Answer from the drawing. Dimensions are ordinates in mm from the lowest x, y and z of the part. A direction names the side the tool comes from. Give positions to 0.01 mm unless a question says otherwise; leave off trailing zeros. Loops run counter-clockwise (first coordinate to the right, second up) from the corner with the lowest first, then second, coordinate; pieces in that order, holes last.
Item 1: A tool of negligible diameter and unlimited length cuts with its end or side. For the marked faces 1 and 2, from which of +Z, -Z, +X, -X, +Y, -Y can it reach the whole face along a straight path? Write none if from no direction.
Item 2: Each of these flat-tipped pins is pushed along its axis until it touches: pin 1 Ø5 at (x, z) = (35.55, 5.32) entering from +Y; pin 2 Ø8 at (x, y) = (52.5, 12) entering from +Z. Where does it stop, or does it pass through?
Item 3: Section D-D, the plane z = 6.5 is taken. Give the vertices of the cut face in (x, y) (1 decimal), and give its area (3 significant figures).
Item 4: Consider line 1 along X through (y, z) = (4, 18.75) (1 decimal); line 2 along Y through (x, z) = (54, 17.25). Determine where each line is inside the solid, lowest interval first.
Item 5: Section A-A, the plane y = 14.5 is taken. Give the vertices of the cut face in (x, z) (1 decimal).
Item 6: Section B-B, the plane z = 15.5 is taken. Give the vertices of the cut face in (x, y) (1 decimal).
Item 7: Section C-C, the plane x = 64 is taken. Give the vertices of the cut face in (y, z).
Item 8: The mould has two halves that part along X. Classify the marked faces 3, 4 and 5: pulls with the +X half, pulls with the -X half, needs draft (parallel to the pull), parting line crosses it, or undercut.
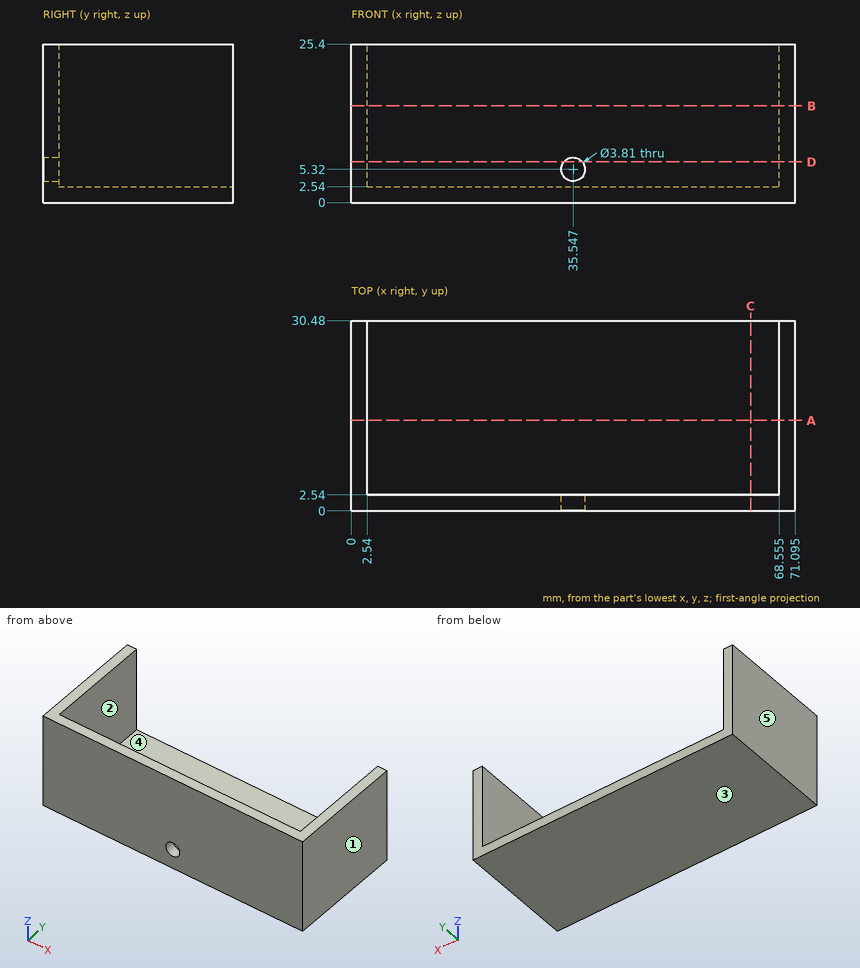
Worked answers:
1. face 1: +Z, -Z, +X, +Y, -Y
1. face 2: +Z, +Y
2. pin 1: stops at y = 2.54
2. pin 2: stops at z = 2.54
3. outline: (0, 0) - (34.1, 0) - (34.1, 2.5) - (2.5, 2.5) - (2.5, 30.5) - (0, 30.5) - close; (37, 0) - (71.1, 0) - (71.1, 30.5) - (68.6, 30.5) - (68.6, 2.5) - (37, 2.5) - close
3. area: 315 mm2
4. line 1: x = 0 to 2.5, 68.6 to 71.1
4. line 2: y = 0 to 2.54
5. outline: (0, 0) - (71.1, 0) - (71.1, 25.4) - (68.6, 25.4) - (68.6, 2.5) - (2.5, 2.5) - (2.5, 25.4) - (0, 25.4) - close
6. outline: (0, 0) - (71.1, 0) - (71.1, 30.5) - (68.6, 30.5) - (68.6, 2.5) - (2.5, 2.5) - (2.5, 30.5) - (0, 30.5) - close
7. outline: (0, 0) - (30.48, 0) - (30.48, 2.54) - (2.54, 2.54) - (2.54, 25.4) - (0, 25.4) - close
8. face 3: needs draft
8. face 4: undercut
8. face 5: pulls with the -X half
